from build123d import *

# Parameters (mm, degrees)
SKETCH1_R           = 11
BOSS_EXTRUDE1_DEPTH = 20
SKETCH2_R           = 8
CUT_EXTRUDE1_DEPTH  = 17
SKETCH3_W           = 10
SKETCH3_H           = 19.595917942
BOSS_EXTRUDE2_DEPTH = 30
SKETCH4_R           = 4
CUT_EXTRUDE2_DEPTH  = 17
FILLET1_R           = 9
CUT_EXTRUDE3_DEPTH  = 51
SKETCH6_R           = 3.15
CUT_EXTRUDE4_DEPTH  = 20.595917942


with BuildPart() as part:
    # Sketch1 → Boss-Extrude1 (new body)
    with BuildSketch(Plane(origin=(0, 0, 0), x_dir=(1, 0, 0), z_dir=(0, 1, 0))):
        Circle(SKETCH1_R)
    extrude(amount=BOSS_EXTRUDE1_DEPTH)

    # Sketch2 → Cut-Extrude1 (cut)
    with BuildSketch(Plane(origin=(0, 20, 0), x_dir=(1, 0, 0), z_dir=(0, 1, 0))):
        Circle(SKETCH2_R)
    extrude(amount=-CUT_EXTRUDE1_DEPTH, mode=Mode.SUBTRACT)

    # Sketch3 → Boss-Extrude2 (add)
    with BuildSketch(Plane.XZ):
        Rectangle(SKETCH3_W, SKETCH3_H)
    extrude(amount=BOSS_EXTRUDE2_DEPTH)

    # Sketch4 → Cut-Extrude2 (cut, through all)
    with BuildSketch(Plane(origin=(5, 0, 0), x_dir=(0, 0, -1), z_dir=(1, 0, 0))):
        with Locations((0, -21)):
            Circle(SKETCH4_R)
    extrude(amount=-CUT_EXTRUDE2_DEPTH, mode=Mode.SUBTRACT)

    # Fillet1
    fillet1_edges = [part.edges().sort_by_distance(p)[0] for p in [
        (0, -30, 9.797958971),
        (0, -30, -9.797958971),
    ]]
    fillet(fillet1_edges, radius=FILLET1_R)

    # Sketch5 → Cut-Extrude3 (cut, through all)
    with BuildSketch(Plane(origin=(0, 20, 0), x_dir=(1, 0, 0), z_dir=(0, 1, 0))):
        with BuildLine():
            Line((-9.797958971, 5), (-9.797958971, -5))
            ThreePointArc((-9.797958971, -5), (-11, 0), (-9.797958971, 5))
        make_face()
        with BuildLine():
            Line((9.797958971, -5), (9.797958971, 5))
            ThreePointArc((9.797958971, 5), (11, 0), (9.797958971, -5))
        make_face()
    extrude(amount=-CUT_EXTRUDE3_DEPTH, mode=Mode.SUBTRACT)

    # Sketch6 → Cut-Extrude4 (cut, through all)
    with BuildSketch(Plane.ZY.offset(9.797958971)):
        with Locations((0, 12.35)):
            Circle(SKETCH6_R)
    extrude(amount=-CUT_EXTRUDE4_DEPTH, mode=Mode.SUBTRACT)


solid = part.part
Design review of the part built by this model. Coordinates are the model's own, in mm. A direction names the side the tool comes from. Give positions to 0.01 mm unless a question says otherwise; leave off trailing zeros. Order: outer loops, then holes, each group sorted by start corner. A loop starts at its lowest first (then second) coordinate and runs counter-clockwise, first axis right, second up. Notation, with made-up numbers: (61, 72) - (91, 72) arc R11 ccw to (91, 85) - close; hole circle Ø4 at (26.5, 34.25). An arc over 180 degrees is marked (long way). Write item = value, one per line. Start each with the question number.
Q1. Mouldability with a two-part tool opening along Y and no side actions: class faces 6 (the face through (8.83, 11.14, 2.91)), 7 (the face through (0.07, -27.294, 7.232)), 8 (the face through (0, -10, 9.798)) as released by +Y, released by -Y, zero draft, split by the parting line, or undercut.
Q2. We need section A-A on y = 12.35. State the section outline as (x, z) points.
Q3. Clearance check with flat-ended pins moving along their axes: pin 1 Ø3 at (y, z) = (4.5, -7) entering from +X; pin 2 Ø1.5 at (y, z) = (-3, 0) entering from +X; pin 3 Ø3 at (x, y) = (0, -15) entering from -Z; pin 4 Ø5 at (y, z) = (12.35, 0) entering from +X. State where each tip first meets the part, or that it passes through.
Q4. We need section C-C on x = 0. State the section outline as (y, z) points.
Q5. To check wall thickness, follow L1, parallel to Y at x = 9.05, z = 0; L2, parallel to Z at x = -0.5, y = -6; L3, parallel to Y at x = 5.5, z = -5.25. State the ranges of each line that lie inside material, in increasing order. Write a range as from..to.
Q6. We need section B-B on z = 0. State the section outline as (x, y) points, plus the area to 3 significant figures.
Q7. We need section D-D on z = 9.25. State the section outline as (x, y) points.
Q8. Tool access review of faces 1 (the face through (7, 0, 0)), 2 (the face through (0, 3, 0)), 3 (the face through (0, 0, 10)), 4 (the face through (-5, -15, 0)), 5 (the face through (0, -10, -9.798)): name each direction out of +Z, -Z, +X, -X, +Y, -Y from which nothing blocks a thin tool from reaching the whole face with its end or side.
Working result:
q1.face_6 = undercut
q1.face_7 = released by -Y
q1.face_8 = zero draft
q2.outline = (-9.8, -5) arc R11 ccw to (9.8, -5) - (9.8, -3.15) - (7.35, -3.15) arc R8 cw to (-7.35, -3.15) - (-9.8, -3.15) - close; (-9.8, 3.15) - (-7.35, 3.15) arc R8 cw to (7.35, 3.15) - (9.8, 3.15) - (9.8, 5) arc R11 ccw to (-9.8, 5) - close
q3.pin_1 = 9.53
q3.pin_2 = 5
q3.pin_3 = -9.8
q3.pin_4 = through
q4.outline = (-30, -0.8) arc R9 ccw to (-21, -9.8) - (0, -9.8) - (0, -11) - (20, -11) - (20, -8) - (3, -8) - (3, 8) - (20, 8) - (20, 11) - (0, 11) - (0, 9.8) - (-21, 9.8) arc R9 ccw to (-30, 0.8) - close; hole circle Ø8 at (-21, 0)
q5.L1 = 0..9.2, 15.5..20
q5.L2 = -9.8..9.8
q5.L3 = 0..3
q6.outline = (-9.8, 0) - (-5, 0) - (-5, -17) - (5, -17) - (5, 0) - (9.8, 0) - (9.8, 9.2) - (8, 9.2) - (8, 3) - (-8, 3) - (-8, 9.2) - (-9.8, 9.2) - close; (-9.8, 15.5) - (-8, 15.5) - (-8, 20) - (-9.8, 20) - close; (-5, -30) - (5, -30) - (5, -25) - (-5, -25) - close; (8, 15.5) - (9.8, 15.5) - (9.8, 20) - (8, 20) - close
q6.area = 317 mm²
q7.outline = (-5.95, 0) - (-5, 0) - (-5, -24.09) - (5, -24.09) - (5, 0) - (5.95, 0) - (5.95, 20) - (-5.95, 20) - close
q8.face_1 = +Z, -Z, +X, -Y
q8.face_2 = +Y
q8.face_3 = +Z, +X, -X, -Y
q8.face_4 = +Z, -Z, -X, -Y
q8.face_5 = -Z, +X, -X, -Y
